from build123d import *

# Parameters (mm, degrees)
SKETCH1_R           = 25.4
BOSS_EXTRUDE1_DEPTH = 76.2
SHELL1_T            = 6.35
CUT_EXTRUDE1_REACH  = 86.242
SKETCH2_R           = 9.525


with BuildPart() as part:
    # Sketch1 → Boss-Extrude1 (new body)
    with BuildSketch(Plane(origin=(0, 0, 0), x_dir=(1, 0, 0), z_dir=(0, 1, 0))):
        with Locations(Location((0, 0, 0), (0, 0, 90))):
            Circle(SKETCH1_R)
    extrude(amount=BOSS_EXTRUDE1_DEPTH)

    # Shell1 (no face opened: a closed hollow body)
    add(offset(amount=-SHELL1_T, mode=Mode.PRIVATE), mode=Mode.SUBTRACT)

    # Sketch2 → Cut-Extrude1 (cut, up to next)
    with BuildSketch(Plane.XZ, mode=Mode.PRIVATE) as cut_extrude1_sk1:
        with Locations(Location((0, 0, 0), (0, 0, 270))):
            Circle(SKETCH2_R)
    cut_extrude1_tool1 = extrude(cut_extrude1_sk1.sketch, amount=-CUT_EXTRUDE1_REACH, mode=Mode.PRIVATE) & part.part
    add(cut_extrude1_tool1.solids().sort_by_distance((0, 0, 0))[0], mode=Mode.SUBTRACT)


solid = part.part
Input: part model. Units: mm. Frame: model coordinates. A direction names the side the tool comes from. Coordinates: 2 decimals unless noted, no trailing zeros. Order: outer loops, then holes, each group sorted by start corner. A loop starts at its lowest first (then second) coordinate and runs counter-clockwise, first axis right, second up. Notation, with made-up numbers: M -37,-35.75 L 7,-35.75 A23 cw 7,-6.75 Z; hole C 32,67 d5. An arc over 180 degrees is marked long. Answer in a Markdown table with one row per item.
(1) Contact query for flat-ended pins moving along their axis: pin 1 Ø2 at (y, z) = (67.5, 18.5) entering from -X; pin 2 Ø3 at (x, y) = (-4.5, 12) entering from -Z; pin 3 Ø4 at (x, y) = (18, 12.5) entering from +Z. Output: stop coordinate, or through.
Numbers:
| item | result |
|---|---|
| pin 1 | stops at x = -18.41 |
| pin 2 | stops at z = -25.22 |
| pin 3 | stops at z = 19.73 |
(2) Section query D-D, the plane z = 15. Output: boundary loops of the cut face in (x, y), plus the area to 3 significant figures.
Numbers:
| item | result |
|---|---|
| outline | M -20.5,0 L 20.5,0 L 20.5,76.2 L -20.5,76.2 Z; hole M -11.74,6.35 L 11.74,6.35 L 11.74,69.85 L -11.74,69.85 Z |
| area | 1,630 mm^2 |
(3) Section query C-C, the plane x = 15. Output: boundary loops of the cut face in (y, z).
Numbers:
| item | result |
|---|---|
| outline | M 0,-20.5 L 76.2,-20.5 L 76.2,20.5 L 0,20.5 Z; hole M 6.35,-11.74 L 69.85,-11.74 L 69.85,11.74 L 6.35,11.74 Z |
(4) Material intervals for line 1 (X direction, y = 32, z = 0); line 2 (Y direction, x = -16.5, z = -1.5); line 3 (X direction, y = 4, z = 0) (3 decimals), sorted ascending. Write a range as [from, to].
Numbers:
| item | result |
|---|---|
| line 1 | x = [-25.4, -19.05], [19.05, 25.4] |
| line 2 | y = [0, 6.35], [69.85, 76.2] |
| line 3 | x = [-25.4, -9.525], [9.525, 25.4] |
(5) Access query for faces 1 (the flat face through (0, 0, -11)), 2 (the flat face through (4, 6.35, 9)). Directions: +Z, -Z, +X, -X, +Y, -Y. A direction counts if a zero-diameter tool reaches every point of the face in a straight line with its end or side. Return the directions, or none.
Numbers:
| item | result |
|---|---|
| face 1 | +Z, -Z, +X, -X, -Y |
| face 2 | none |
(6) Section query A-A, the plane x = 0. Output: boundary loops of the cut face in (y, z) (3 decimals).
Numbers:
| item | result |
|---|---|
| outline | M 0,-25.4 L 76.2,-25.4 L 76.2,25.4 L 0,25.4 L 0,9.525 L 6.35,9.525 L 6.35,19.05 L 69.85,19.05 L 69.85,-19.05 L 6.35,-19.05 L 6.35,-9.525 L 0,-9.525 Z |
(7) Section query B-B, the plane z = 0. Output: boundary loops of the cut face in (x, y) (3 decimals), plus the area to 3 significant figures.
Numbers:
| item | result |
|---|---|
| outline | M -25.4,0 L -9.525,0 L -9.525,6.35 L -19.05,6.35 L -19.05,69.85 L 19.05,69.85 L 19.05,6.35 L 9.525,6.35 L 9.525,0 L 25.4,0 L 25.4,76.2 L -25.4,76.2 Z |
| area | 1,330 mm^2 |
(8) Draft query along Y for faces 3 (the cylindrical face through (-5.796, 3.131, 7.559)), 4 (the flat face through (0, 69.85, 0)), 5 (the flat face through (0, 76.2, 0)). Return one class per face: pulls with the +Y half, pulls with the -Y half, needs draft (parallel to the pull), parting line crosses it, or undercut.
Numbers:
| item | result |
|---|---|
| face 3 | needs draft |
| face 4 | undercut |
| face 5 | pulls with the +Y half |
